from build123d import *

# Parameters (mm, degrees)
ESQUISSE1_W             = 121.6
ESQUISSE1_H             = 65.9
BOSS_EXTRU_1_DEPTH      = 1.5
CONG_1_R                = 3
ESQUISSE2_R             = 1.7
ENL_V_MAT_EXTRU_1_DEPTH = 70.170748876


with BuildPart() as part:
    # Esquisse1 → Boss.-Extru.1 (new body)
    with BuildSketch(Plane(origin=(0, 0, 0), x_dir=(1, 0, 0), z_dir=(0, 1, 0))):
        Rectangle(ESQUISSE1_W, ESQUISSE1_H)
    extrude(amount=BOSS_EXTRU_1_DEPTH)

    # Congé1
    cong_1_edges = [part.edges().sort_by_distance(p)[0] for p in [
        (60.8, 0.75, 32.95),
        (-60.8, 0.75, 32.95),
        (-60.8, 0.75, -32.95),
        (60.8, 0.75, -32.95),
    ]]
    fillet(cong_1_edges, radius=CONG_1_R)

    # Esquisse2 → Enlèv. mat.-Extru.1 (cut, through all)
    with BuildSketch(Plane(origin=(0, 1.5, 0), x_dir=(1, 0, 0), z_dir=(0, 1, 0))):
        with Locations(Location((-56.75, 28.45, 0), (0, 0, 270))):
            Circle(ESQUISSE2_R)
        with Locations(Location((-56.75, 3.25, 0), (0, 0, 270))):
            Circle(ESQUISSE2_R)
        with Locations(Location((56.75, 28.45, 0), (0, 0, 270))):
            Circle(ESQUISSE2_R)
        with Locations(Location((56.75, 3.25, 0), (0, 0, 270))):
            Circle(ESQUISSE2_R)
    extrude(amount=-ENL_V_MAT_EXTRU_1_DEPTH, mode=Mode.SUBTRACT)


solid = part.part
Model file for the job. Use its own axes, mm. Give positions to 0.01 mm unless a question says otherwise; leave off trailing zeros. Loops run counter-clockwise (first coordinate to the right, second up) from the corner with the lowest first, then second, coordinate; pieces in that order, holes last.
Item 1: Drill centre lines: line 1 along X through (y, z) = (0.45, -28.45); line 2 along X through (y, z) = (0.8, -30). Where is each one in solid material? Low to high.
Check values:
line 1: x = -60.8 to -58.45, -55.05 to 55.05, 58.45 to 60.8
line 2: x = -60.8 to -57.45, -56.05 to 56.05, 57.45 to 60.8
Item 2: Slice it at A-A (z = -3.25). Write the cut outline in (x, y).
Check values:
outline: (-60.8, 0) - (-58.45, 0) - (-58.45, 1.5) - (-60.8, 1.5) - close; (-55.05, 0) - (55.05, 0) - (55.05, 1.5) - (-55.05, 1.5) - close; (58.45, 0) - (60.8, 0) - (60.8, 1.5) - (58.45, 1.5) - close
Item 3: Mould opens along X. For faces 1 (the face through (58.183, 0.76, -2.336)), 2 (the face through (-59.94, 0.76, -32.05)), 3 (the face through (59.94, 0.76, -32.05)) say: +X half, -X half, draft (parallel to the pull), parting line (faces both ways), or undercut.
Check values:
face 1: undercut
face 2: -X half
face 3: +X half
